For this review, take the finished solid that the model builds, in its own axes (mm). A direction names the side the tool comes from. Give positions to 0.01 mm unless a question says otherwise; leave off trailing zeros. Write each loop counter-clockwise with the first axis right and the second up, starting at its lowest first coordinate (ties: lowest second). Pieces come first, ordered by that corner, then holes. Notation, with made-up numbers: M 23.5,40.5 L 74.5,40.5 A17 cw 74.5,57.5 Z; hole C 49,55 d7. An arc over 180 degrees is marked long. Use one line per item in the form item = value. Start each with the question number.
Q1. Consider section D-D on z = 6.5. Write out the cut boundary in (x, y), and give its area (3 significant figures).
Q2. Clearance check with flat-ended pins moving along their axes: pin 1 Ø2.5 at (x, y) = (-6.73, 0) entering from +Z; pin 2 Ø1.3 at (x, y) = (-6, -0.5) entering from -Z; pin 3 Ø8 at (y, z) = (-7, 16.5) entering from -X. State where each tip first meets the part, or that it passes through.
Q3. Mouldability with a two-part tool opening along X and no side actions: class faces 4 (the cylindrical face through (-0.205, 1.564, 28.86)), 5 (the flat face through (0, 10, 0.063)), 6 (the flat face through (0, 0, -4.356)) as released by +X, released by -X, zero draft, split by the parting line, or undercut.
Q4. Consider section C-C on z = 29. Write out the cut boundary in (x, y).
Q5. For probe 1 along Y at (x, z) = (0, -2.5) (3 decimals); probe 2 along X at (y, z) = (0, -1.45); probe 3 along Z at (x, y) = (-0.5, -9), list the stretches that pass through material, from the lowest coordinate up. Write a range as [from, to].
Q6. Tool access review of faces 1 (the cylindrical face through (-0.275, -8.285, -1.546)), 2 (the flat face through (0, -2, 22.962)), 3 (the cylindrical face through (-3.004, -13.526, 9.135)): name each direction out of +Z, -Z, +X, -X, +Y, -Y from which nothing blocks a thin tool from reaching the whole face with its end or side.
```python
from build123d import *

# Parameters (mm, degrees)
SKETCH_R     = 13.8557
PAD_DEPTH    = 18.3515
SKETCH001_R  = 12.55395
PAD001_DEPTH = 3.1115
SKETCH002_R  = 13.8557
PAD002_DEPTH = 2.7178
CHAMFER_SIZE = 2.54
SKETCH003_R  = 4.69265
PAD003_DEPTH = 1.8923
SKETCH004_R  = 1.57734
PAD004_DEPTH = 11.9634
SKETCH005_R  = 1.27
POCKET_DEPTH = 3.175
SKETCH006_R  = 1.5875
PAD005_DEPTH = 1.2446


with BuildPart() as part:
    # Sketch → Pad (new body)
    with BuildSketch(Plane.XY):
        Circle(SKETCH_R)
    extrude(amount=PAD_DEPTH)

    # Sketch001 → Pad001 (new body)
    with BuildSketch(Plane(origin=(0, 0, 0), x_dir=(1, 0, 0), z_dir=(0, 0, -1))):
        Circle(SKETCH001_R)
    extrude(amount=PAD001_DEPTH)

    # Sketch002 → Pad002 (new body)
    with BuildSketch(Plane.XY.offset(18.3515)):
        Circle(SKETCH002_R)
    extrude(amount=PAD002_DEPTH)

    # Chamfer
    chamfer_edges = [part.edges().sort_by_distance(p)[0] for p in [
        (-13.8557, 0, 21.0693),
    ]]
    chamfer(chamfer_edges, length=CHAMFER_SIZE)

    # Sketch003 → Pad003 (new body)
    with BuildSketch(Plane.XY.offset(21.0693)):
        Circle(SKETCH003_R)
    extrude(amount=PAD003_DEPTH)

    # Sketch004 → Pad004 (new body)
    with BuildSketch(Plane.XY.offset(22.9616)):
        Circle(SKETCH004_R)
    extrude(amount=PAD004_DEPTH)

    # Sketch005 → Pocket (cut)
    with BuildSketch(Plane(origin=(0, 0, -3.1115), x_dir=(1, 0, 0), z_dir=(0, 0, -1))):
        with Locations((6.73354, 0)):
            Circle(SKETCH005_R)
        with Locations((-6.73354, 0)):
            Circle(SKETCH005_R)
        with Locations((0, 9.525)):
            Circle(SKETCH005_R)
        with Locations((0, -9.525)):
            Circle(SKETCH005_R)
    extrude(amount=-POCKET_DEPTH, mode=Mode.SUBTRACT)

    # Sketch006 → Pad005 (new body)
    with BuildSketch(Plane(origin=(0, 0, -3.1115), x_dir=(1, 0, 0), z_dir=(0, 0, -1))):
        Circle(SKETCH006_R)
    extrude(amount=PAD005_DEPTH)


solid = part.part
```
Working result:
q1.outline = C 0,0 d27.71
q1.area = 603 mm²
q2.pin_1 = 21.07
q2.pin_2 = -3.11
q2.pin_3 = -13.53
q3.face_4 = split by the parting line
q3.face_5 = undercut
q3.face_6 = zero draft
q4.outline = C 0,0 d3.15
q5.probe_1 = [-12.554, -10.795], [-8.255, 8.255], [10.795, 12.554]
q5.probe_2 = [-12.55, -8], [-5.46, 5.46], [8, 12.55]
q5.probe_3 = [0.06, 21.07]
q6.face_1 = -Z
q6.face_2 = +Z
q6.face_3 = +Z, -Z
